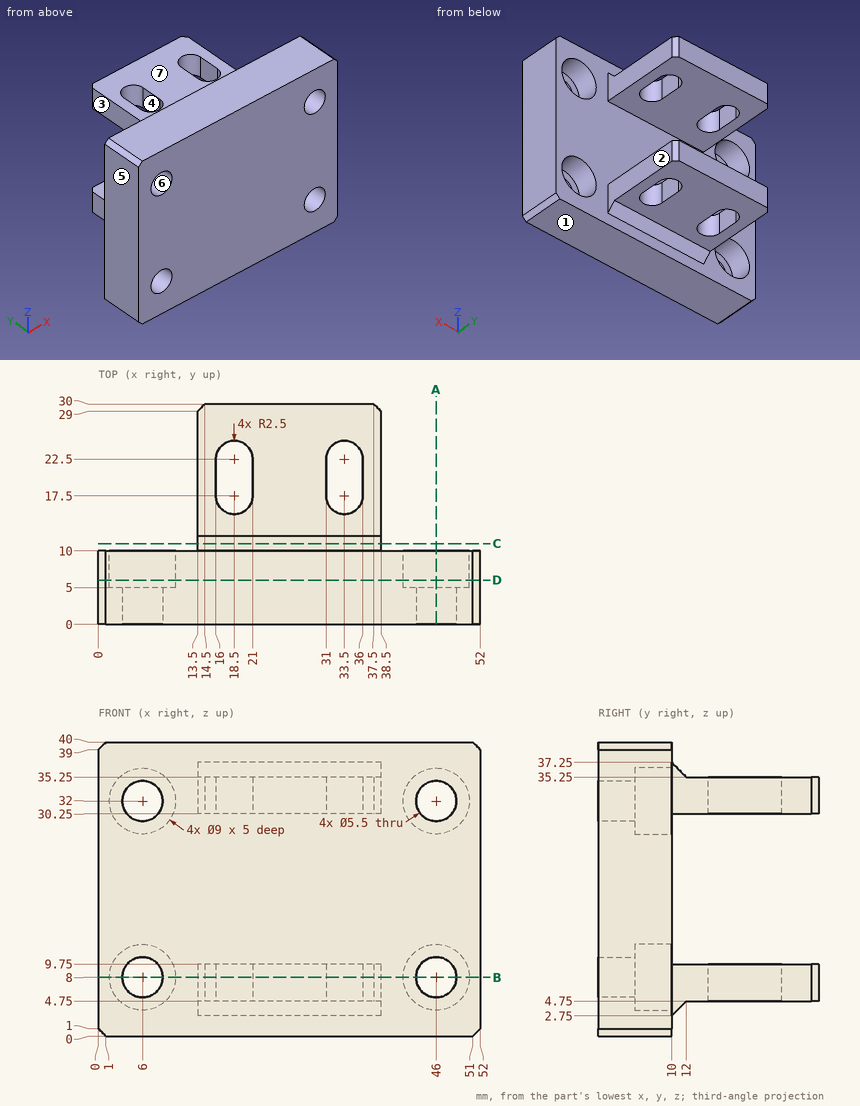
Answer from the drawing. Dimensions are ordinates in mm from the lowest x, y and z of the part. A direction names the side the tool comes from. Give positions to 0.01 mm unless a question says otherwise; leave off trailing zeros. Loops run counter-clockwise (first coordinate to the right, second up) from the corner with the lowest first, then second, coordinate; pieces in that order, holes last. Notation, with made-up numbers: (12, 11) -> (51, 11) arc R20 cw to (51, 50) -> close; hole circle Ø2 at (74.25, -3). An arc over 180 degrees is marked (long way). One line per question, with ' | ' between items. Start each with the question number.
1) Straight lines are drawn through the part: L1, parallel to X at y = 19.5, z = 33.5; L2, parallel to X at y = 6.3, z = 8; L3, parallel to Z at x = 6, y = 1.15. For each, find the intervals that lie inside material, in ascending order.
2) Determine the mould class of the marked faces 5, 6 and 7 for opening direction X: +X half, -X half, draft (parallel to the pull), parting line (faces both ways), or undercut.
3) Section C-C, the plane y = 11 is taken. Determine the outline of the cut face in (x, z).
4) For the marked faces 1, 2, 3 and 4, determine the directions among +Z, -Z, +X, -X, +Y, -Y from which every point of the face is accessible in a straight line to the end or side of a thin tool.
5) Section B-B, the plane z = 8 is taken. State how many separate pieces and enclosed holes the cut face has, then the cut area to 3 significant figures.
6) Section A-A, the plane x = 46 is taken. Determine the outline of the cut face in (y, z), then the cut area to 3 significant figures.
7) Each of these flat-tipped pins is pushed along its axis until it touches: pin 1 (2 mm diameter, centred on x = 35, y = 12, fed in from +Z); pin 2 (6 mm diameter, centred on x = 43, z = 14, fed in from +Y); pin 3 (2 mm diameter, centred on y = 21.5, z = 32.5, fed in from -X); pin 4 (6.5 mm diameter, centred on x = 6, z = 8, fed in from -Y). Where does it stop, or does it pass through?
8) Section D-D, the plane y = 6 is taken. Determine the outline of the cut face in (x, z), then the cut area to 3 significant figures.
Resolved:
1) L1: 13.5 to 16, 21 to 31, 36 to 38.5 | L2: 0 to 1.5, 10.5 to 41.5, 50.5 to 52 | L3: 0 to 5.25, 10.75 to 29.25, 34.75 to 40
2) face 5: -X half | face 6: undercut | face 7: draft
3) outline: (13.5, 3.75) -> (38.5, 3.75) -> (38.5, 9.75) -> (13.5, 9.75) -> close; (13.5, 30.25) -> (38.5, 30.25) -> (38.5, 36.25) -> (13.5, 36.25) -> close
4) face 1: -Z, +X, -X, +Y, -Y | face 2: +Z, -Z, +X, +Y | face 3: +Z, -Z, -X, +Y | face 4: +Z, -Z
5) separate pieces: 3 | enclosed holes: 2 | area: 785 mm2
6) outline: (0, 0) -> (10, 0) -> (10, 3.5) -> (5, 3.5) -> (5, 5.25) -> (0, 5.25) -> close; (0, 10.75) -> (5, 10.75) -> (5, 12.5) -> (10, 12.5) -> (10, 27.5) -> (5, 27.5) -> (5, 29.25) -> (0, 29.25) -> close; (0, 34.75) -> (5, 34.75) -> (5, 36.5) -> (10, 36.5) -> (10, 40) -> (0, 40) -> close | area: 255 mm2
7) pin 1: z = 36.25 | pin 2: y = 10 | pin 3: x = 13.5 | pin 4: y = 0
8) outline: (0, 1) -> (1, 0) -> (51, 0) -> (52, 1) -> (52, 39) -> (51, 40) -> (1, 40) -> (0, 39) -> close; hole circle Ø9 at (6, 8); hole circle Ø9 at (6, 32); hole circle Ø9 at (46, 8); hole circle Ø9 at (46, 32) | area: 1,820 mm2
